Build history of the part. All positions in model axes, mm. Face numbers are marked on the shaded views. A direction names the side the tool comes from. Round coordinates to 2 decimals unless told otherwise and drop trailing zeros. Write each loop counter-clockwise with the first axis right and the second up, starting at its lowest first coordinate (ties: lowest second). Pieces come first, ordered by that corner, then holes. Notation, with made-up numbers: (2, -29) -> (23, -29) arc R6 cw to (23, -24) -> close; hole circle Ø8 at (-17, 1.25). An arc over 180 degrees is marked (long way). Return JSON: item names as keys, results as strings.
from build123d import *

# Parameters (mm, degrees)
SKETCH1_W           = 80
SKETCH1_H           = 80
SKETCH1_R           = 36.5
SKETCH1_R_2         = 35
BOSS_EXTRUDE3_DEPTH = 2
BOSS_EXTRUDE4_START = 50
SKETCH1_7_R         = 36.5
SKETCH1_7_R_2       = 35
BOSS_EXTRUDE4_DEPTH = 50
BOSS_EXTRUDE5_DEPTH = 77.35
SKETCH4_R           = 36
BOSS_EXTRUDE6_DEPTH = 1.5


with BuildPart() as part:
    # Sketch1 → Boss-Extrude3 (new body)
    # profile 1 of 2: a face of its own
    with BuildSketch(Plane(origin=(0, 0, 0), x_dir=(1, 0, 0), z_dir=(0, 1, 0))):
        Rectangle(SKETCH1_W, SKETCH1_H)
        Circle(SKETCH1_R, mode=Mode.SUBTRACT)
    # profile 2 of 2: a face of its own
    with BuildSketch(Plane(origin=(0, 0, 0), x_dir=(1, 0, 0), z_dir=(0, 1, 0))):
        Circle(SKETCH1_R)
        with Locations(Location((0, 0, 0), (0, 0, 270))):
            Circle(SKETCH1_R_2, mode=Mode.SUBTRACT)
    extrude(amount=-BOSS_EXTRUDE3_DEPTH)

    # Sketch1<7> → Boss-Extrude4 (add)
    with BuildSketch(Plane(origin=(0, 0, 0), x_dir=(1, 0, 0), z_dir=(0, 1, 0)).offset(BOSS_EXTRUDE4_START)):
        with Locations(Location((0, 0, 0), (0, 0, 270))):
            Circle(SKETCH1_7_R)
        with Locations(Location((0, 0, 0), (0, 0, 270))):
            Circle(SKETCH1_7_R_2, mode=Mode.SUBTRACT)
    extrude(amount=-BOSS_EXTRUDE4_DEPTH)

    # Sketch3 → Boss-Extrude5 (add)
    with BuildSketch(Plane.XY.offset(40)):
        Polygon((-32.3, -2), (-34.8, -2), (-34.8, -4.3), (-37.3, -4.3), (-37.3, -6.3), (-32.3, -6.3), align=None)
        Polygon((32.3, -6.3), (37.3, -6.3), (37.3, -4.3), (34.8, -4.3), (34.8, -2), (32.3, -2), align=None)
    extrude(amount=-BOSS_EXTRUDE5_DEPTH)

    # Sketch4 → Boss-Extrude6 (add)
    with BuildSketch(Plane(origin=(0, 50, 0), x_dir=(1, 0, 0), z_dir=(0, 1, 0))):
        Circle(SKETCH4_R)
    extrude(amount=-BOSS_EXTRUDE6_DEPTH)


solid = part.part
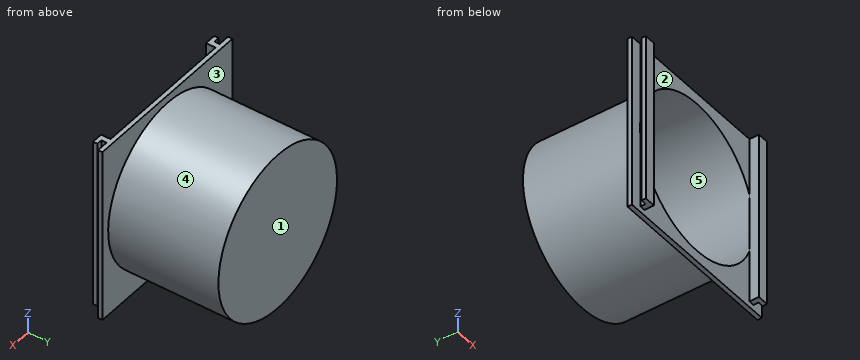
Q1. Wall check: L1, parallel to Y at x = -33.5, z = 7; L2, parallel to Y at x = 37, z = -17; L3, parallel to X at y = 22, z = 0. Give the ranges that are in metal, low to high.
Verdict:
{"L1": "y = -6.3 to -2, 48.5 to 50", "L2": "y = -6.3 to -4.3, -2 to 0", "L3": "x = -36.5 to -35, 35 to 36.5"}
Q2. Two-plate mould, pull along X, no slides. Class the marked faces 3, 4 and 5: +X half, -X half, draft (parallel to the pull), parting line (faces both ways), or undercut.
Verdict:
{"face 3": "draft", "face 4": "parting line", "face 5": "undercut"}
Q3. Saw through at D-D on x = -12. List the corners of the cut face in (y, z).
Verdict:
{"outline": "(-2, -40) -> (0, -40) -> (0, -34.47) -> (50, -34.47) -> (50, 34.47) -> (0, 34.47) -> (0, 40) -> (-2, 40) -> (-2, 32.88) -> (48.5, 32.88) -> (48.5, -32.88) -> (-2, -32.88) -> close"}
Q4. Saw through at B-B on x = 0. List the corners of the cut face in (y, z).
Verdict:
{"outline": "(-2, -40) -> (0, -40) -> (0, -36.5) -> (50, -36.5) -> (50, 36.5) -> (0, 36.5) -> (0, 40) -> (-2, 40) -> (-2, 35) -> (48.5, 35) -> (48.5, -35) -> (-2, -35) -> close"}
Q5. 3-axis set-ups, long thin cutter, end or side, ignore diameter. For the marked faces 1 and 2: which of +Z, -Z, +X, -X, +Y, -Y reach the whole face in a straight line?
Verdict:
{"face 1": "+Z, -Z, +X, -X, +Y", "face 2": "+Z, -Z, -Y"}
Q6. Pin check, flat tips, straight feed: pin 1 Ø12 at (x, y) = (-30, 22) entering from -Z; pin 2 Ø1 at (y, z) = (-5, 14.5) entering from +X; pin 3 Ø6 at (x, y) = (-25, 6) entering from +Z. Stop position of each tip, or through.
Verdict:
{"pin 1": "stops at z = -27.5", "pin 2": "stops at x = 37.3", "pin 3": "stops at z = 29.12"}
Q7. Saw through at C-C on y = 31.5. List the corners of the cut face in (x, z).
Verdict:
{"outline": "circle Ø73 at (0, 0); hole circle Ø70 at (0, 0)"}
Q8. Saw through at A-A on z = 0. List the corners of the cut face in (x, y), then the cut area to 4 significant figures.
Verdict:
{"outline": "(-40, -2) -> (-35, -2) -> (-35, 48.5) -> (35, 48.5) -> (35, -2) -> (40, -2) -> (40, 0) -> (36.5, 0) -> (36.5, 50) -> (-36.5, 50) -> (-36.5, 0) -> (-40, 0) -> close; (-37.3, -6.3) -> (-32.3, -6.3) -> (-32.3, -2) -> (-34.8, -2) -> (-34.8, -4.3) -> (-37.3, -4.3) -> close; (32.3, -6.3) -> (37.3, -6.3) -> (37.3, -4.3) -> (34.8, -4.3) -> (34.8, -2) -> (32.3, -2) -> close", "area": "306.5 mm²"}
